Source: CAD feature listing. Evaluate the final solid. Frame: model axes, mm. Face numbers are marked on the shaded views. Round coordinates to 2 decimals unless told otherwise and drop trailing zeros. Order: outer loops, then holes, each group sorted by start corner. A loop starts at its lowest first (then second) coordinate and runs counter-clockwise, first axis right, second up. Notation, with made-up numbers: (43.25, 61) -> (68.25, 61) arc R31 ccw to (68.25, 98) -> close; hole circle Ø1 at (37.5, 45.25). An arc over 180 degrees is marked (long way). Answer as CSV lines item,"result".
from build123d import *

# Parameters (mm, degrees)
SKETCH1_W                   = 76.2
SKETCH1_H                   = 35.56
SKETCH1_R                   = 3.3734375
BOSS_EXTRUDE1_DEPTH         = 21.59
FILLET1_R                   = 6.35
F_1_4_20_TAPPED_HOLE1_D     = 5.1054
F_1_4_20_TAPPED_HOLE1_DEPTH = 26.67
F_1_4_20_TAPPED_HOLE1_TIP   = 1.533816902


with BuildPart() as part:
    # Sketch1 → Boss-Extrude1 (new body)
    with BuildSketch(Plane.XY):
        with Locations((38.1, 17.78)):
            Rectangle(SKETCH1_W, SKETCH1_H)
        with Locations((25.4, 14.478)):
            Circle(SKETCH1_R, mode=Mode.SUBTRACT)
        with Locations((50.8, 14.478)):
            Circle(SKETCH1_R, mode=Mode.SUBTRACT)
    extrude(amount=BOSS_EXTRUDE1_DEPTH)

    # Fillet1
    fillet1_edges = [part.edges().sort_by_distance(p)[0] for p in [
        (0, 0, 10.795),
        (0, 35.56, 10.795),
        (76.2, 35.56, 10.795),
        (76.2, 0, 10.795),
    ]]
    fillet(fillet1_edges, radius=FILLET1_R)

    # 1/4-20 Tapped Hole1
    with Locations(Plane(origin=(0, 25.4, 10.795), x_dir=(0, 0, -1), z_dir=(-1, 0, 0))):
        with Locations((0, 0)):
            Hole(F_1_4_20_TAPPED_HOLE1_D / 2, depth=F_1_4_20_TAPPED_HOLE1_DEPTH)
            with Locations((0, 0, -(F_1_4_20_TAPPED_HOLE1_DEPTH + F_1_4_20_TAPPED_HOLE1_TIP / 2))):  # 118° drill point
                Cone(0, F_1_4_20_TAPPED_HOLE1_D / 2, F_1_4_20_TAPPED_HOLE1_TIP, mode=Mode.SUBTRACT)


solid = part.part
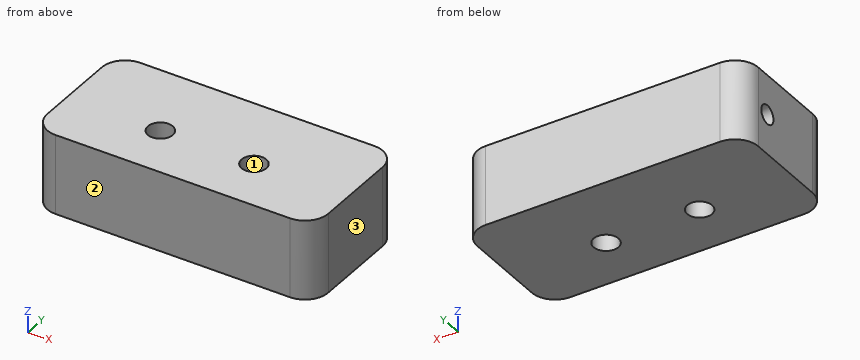
1. Section query A-A on x = 25.4. Return loops of the section in (y, z) (3 decimals).
Results below:
outline,"(0, 0) -> (11.105, 0) -> (11.105, 21.59) -> (0, 21.59) -> close; (17.851, 0) -> (35.56, 0) -> (35.56, 21.59) -> (17.851, 21.59) -> close; hole circle Ø5.105 at (25.4, 10.795)"
2. Section query B-B on z = 6. Return loops of the section in (x, y).
Results below:
outline,"(0, 6.35) arc R6.35 ccw to (6.35, 0) -> (69.85, 0) arc R6.35 ccw to (76.2, 6.35) -> (76.2, 29.21) arc R6.35 ccw to (69.85, 35.56) -> (6.35, 35.56) arc R6.35 ccw to (0, 29.21) -> close; hole circle Ø6.75 at (25.4, 14.48); hole circle Ø6.75 at (50.8, 14.48)"
3. Pin query (flat end, axial travel): pin 1 (5.5 mm diameter, centred on x = 50.8, y = 14.478, fed in from -Z). Return the tip coordinate at first contact, or that it passes through.
Results below:
pin 1,"through"
4. Mould query, pull axis X, two halves, no side actions, for the marked faces 1, 2 and 3. Classes: released by +X, released by -X, zero draft, split by the parting line, or undercut.
Results below:
face 1,"undercut"
face 2,"zero draft"
face 3,"released by +X"
5. Line query: L1, parallel to Y at x = 50.5, z = 17; L2, parallel to Y at x = 50.8, z = 14; L3, parallel to X at y = 15, z = 20. Output: solid intervals per line, ascending. Write a range as [from, to].
Results below:
L1,"[0, 11.12], [17.84, 35.56]"
L2,"[0, 11.1], [17.85, 35.56]"
L3,"[0, 22.07], [28.73, 47.47], [54.13, 76.2]"
6. Section query C-C on x = 50.8. Return loops of the section in (y, z), and give its area (3 significant figures).
Results below:
outline,"(0, 0) -> (11.1, 0) -> (11.1, 21.59) -> (0, 21.59) -> close; (17.85, 0) -> (35.56, 0) -> (35.56, 21.59) -> (17.85, 21.59) -> close"
area,"622 mm2"
